For this review, take the finished solid that the model builds, in its own axes (mm). Face numbers are marked on the shaded views. A direction names the side the tool comes from. Coordinates: 2 decimals unless noted, no trailing zeros. Loops run counter-clockwise (first coordinate to the right, second up) from the corner with the lowest first, then second, coordinate; pieces in that order, holes last. Notation, with made-up numbers: (-28, -25.5) -> (-11, -25.5) arc R18 ccw to (-11, 7.5) -> close; hole circle Ø10 at (-1, 72.25). An arc over 180 degrees is marked (long way). Answer in a Markdown table with one row per item.
from build123d import *

# Parameters (mm, degrees)
Y_KSEKLIK_EKSTR_ZYON1_DEPTH = 12
Y_KSEKLIK_EKSTR_ZYON3_DEPTH = 15
KES_EKSTR_ZYON2_DEPTH       = 10
IZIM7_R                     = 3.5
KES_EKSTR_ZYON3_DEPTH       = 10
IZIM9_W                     = 16.31
IZIM9_H                     = 31
Y_KSEKLIK_EKSTR_ZYON4_DEPTH = 2
IZIM11_W                    = 16.312144578
IZIM11_H                    = 31
Y_KSEKLIK_EKSTR_ZYON5_DEPTH = 2
IZIM12_W                    = 16.312144578
IZIM12_H                    = 2
Y_KSEKLIK_EKSTR_ZYON6_DEPTH = 5
IZIM13_W                    = 16.31
IZIM13_H                    = 2
Y_KSEKLIK_EKSTR_ZYON7_DEPTH = 5
IZIM16_R                    = 1.5
KES_EKSTR_ZYON4_DEPTH       = 5


with BuildPart() as part:
    # Çizim1 → Yükseklik-Ekstrüzyon1 (new body)
    with BuildSketch(Plane(origin=(0, 0, 0), x_dir=(1, 0, 0), z_dir=(0, 1, 0))):
        with BuildLine():
            Line((-10.273080285, 9.233441174), (-24.270017386, 9.23050626))
            ThreePointArc((-24.270017386, 9.23050626), (-27.573247243, 1.740187513), (-24.270017386, -5.750131234))
            ThreePointArc((-24.270017386, -5.750131234), (-24.266862702, -5.754522055), (-24.265747955, -5.759812487))
            Line((-24.265747955, -5.759812487), (-10.280448773, -5.759812487))
            ThreePointArc((-10.280448773, -5.759812487), (-10.279708775, -5.756150024), (-10.277604879, -5.753062168))
            ThreePointArc((-10.277604879, -5.753062168), (-7.119784217, 1.739236804), (-10.273080285, 9.233441174))
        make_face()
    extrude(amount=Y_KSEKLIK_EKSTR_ZYON1_DEPTH)

    # Çizim2 → Yükseklik-Ekstrüzyon3 (add)
    with BuildSketch(Plane(origin=(0, 12, 0), x_dir=(1, 0, 0), z_dir=(0, 1, 0))):
        Polygon((-28.472879545, -6.371596623), (-24.972879545, -6.371596623), (-6.065973504, -6.371596623), (-6.065973504, 9.940547955), (-9.565973504, 9.940547955), (-28.472879545, 9.940547955), align=None)
        with BuildLine():
            ThreePointArc((-10.277604879, -5.753062168), (-10.279708775, -5.756150024), (-10.280448773, -5.759812487))
            Line((-10.280448773, -5.759812487), (-24.265747955, -5.759812487))
            ThreePointArc((-24.265747955, -5.759812487), (-24.266862702, -5.754522055), (-24.270017386, -5.750131234))
            ThreePointArc((-24.270017386, -5.750131234), (-27.573247243, 1.740187513), (-24.270017386, 9.23050626))
            Line((-24.270017386, 9.23050626), (-10.273080285, 9.233441174))
            ThreePointArc((-10.273080285, 9.233441174), (-7.119784217, 1.739236804), (-10.277604879, -5.753062168))
        make_face(mode=Mode.SUBTRACT)
    extrude(amount=-Y_KSEKLIK_EKSTR_ZYON3_DEPTH)

    # Çizim5 → Kes-Ekstrüzyon2 (cut)
    with BuildSketch(Plane(origin=(0, 0, 0), x_dir=(1, 0, 0), z_dir=(0, 1, 0))):
        with BuildLine():
            ThreePointArc((-24.253497742, -5.732043117), (-24.24760022, -5.74025453), (-24.24552089, -5.750148186))
            Line((-24.24552089, -5.750148186), (-10.281129786, -5.759812016))
            ThreePointArc((-10.281129786, -5.759812016), (-10.28107446, -5.75954361), (-10.280917812, -5.759318746))
            ThreePointArc((-10.280917812, -5.759318746), (-7.055942633, 1.738860839), (-10.261152425, 9.245510703))
            ThreePointArc((-10.261152425, 9.245510703), (-10.261308072, 9.245735025), (-10.261363099, 9.246002453))
            Line((-10.261363099, 9.246002453), (-24.245520899, 9.230533357))
            ThreePointArc((-24.245520899, 9.230533357), (-24.247598176, 9.220634198), (-24.253497742, 9.212418143))
            ThreePointArc((-24.253497742, 9.212418143), (-27.548750741, 1.740187513), (-24.253497742, -5.732043117))
        make_face()
    extrude(amount=KES_EKSTR_ZYON2_DEPTH, mode=Mode.SUBTRACT)

    # Çizim7 → Kes-Ekstrüzyon3 (cut)
    with BuildSketch(Plane(origin=(0, 12, 0), x_dir=(1, 0, 0), z_dir=(0, 1, 0))):
        with Locations((-17.269426524, 1.784475666)):
            Circle(IZIM7_R)
    extrude(amount=-KES_EKSTR_ZYON3_DEPTH, mode=Mode.SUBTRACT)

    # Çizim9 → Yükseklik-Ekstrüzyon4 (add)
    with BuildSketch(Plane.ZY.offset(28.472879545)):
        with Locations((-1.785547955, -3.5)):
            Rectangle(IZIM9_W, IZIM9_H)
    extrude(amount=Y_KSEKLIK_EKSTR_ZYON4_DEPTH)

    # Çizim11 → Yükseklik-Ekstrüzyon5 (add)
    with BuildSketch(Plane(origin=(-6.065973504, 0, 0), x_dir=(0, 0, -1), z_dir=(1, 0, 0))):
        with Locations((1.784475666, -3.5)):
            Rectangle(IZIM11_W, IZIM11_H)
    extrude(amount=Y_KSEKLIK_EKSTR_ZYON5_DEPTH)

    # Çizim12 → Yükseklik-Ekstrüzyon6 (add)
    with BuildSketch(Plane(origin=(-4.065973504, 0, 0), x_dir=(0, 0, -1), z_dir=(1, 0, 0))):
        with Locations((1.784475666, -18)):
            Rectangle(IZIM12_W, IZIM12_H)
    extrude(amount=Y_KSEKLIK_EKSTR_ZYON6_DEPTH)

    # Çizim13 → Yükseklik-Ekstrüzyon7 (add)
    with BuildSketch(Plane.ZY.offset(30.472879545)):
        with Locations((-1.785547955, -18)):
            Rectangle(IZIM13_W, IZIM13_H)
    extrude(amount=Y_KSEKLIK_EKSTR_ZYON7_DEPTH)

    # Çizim16 → Kes-Ekstrüzyon4 (cut)
    with BuildSketch(Plane.XZ.offset(19)):
        with Locations((-32.472879545, -1.785547955)):
            Circle(IZIM16_R)
        with Locations((-2.065973504, -1.784475666)):
            Circle(IZIM16_R)
    extrude(amount=-KES_EKSTR_ZYON4_DEPTH, mode=Mode.SUBTRACT)


solid = part.part
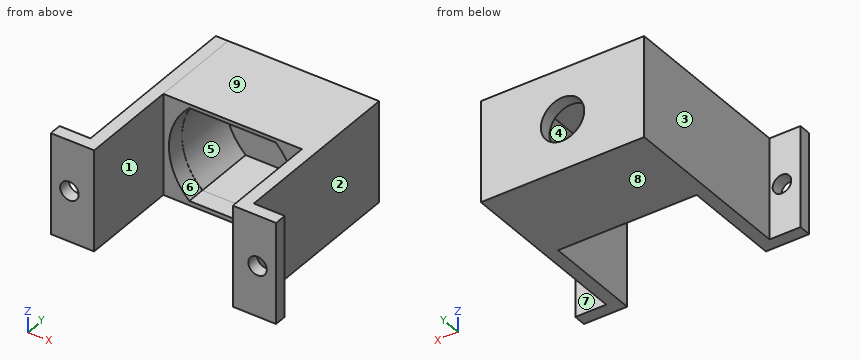
Item 1: Take a section at A-A, the plane y = -11.5. State the section outline as (x, z) points.
Worked answers:
| item | result |
|---|---|
| outline | (-30.47, -9.94) -> (-28.47, -9.94) -> (-28.47, 6.37) -> (-30.47, 6.37) -> close; (-6.07, -9.94) -> (-4.07, -9.94) -> (-4.07, 6.37) -> (-6.07, 6.37) -> close |
Item 2: For L1, parallel to X at y = -14, z = 4.25; L2, parallel to Z at x = -30, y = -1.5; L3, parallel to Y at x = -24, z = -1.25, list the stretches that pass through material, from the lowest coordinate up.
Worked answers:
| item | result |
|---|---|
| L1 | -30.47 to -28.47, -6.07 to -4.07 |
| L2 | -9.94 to 6.37 |
| L3 | 10 to 12 |
Item 3: Insertion check: pin 1 (6 mm diameter, centred on y = 6, z = 4.5, fed in from +X); pin 2 (8 mm diameter, centred on x = -11.5, z = -1.5, fed in from -Y); pin 3 (8 mm diameter, centred on y = -14, z = 1.5, fed in from -X); pin 4 (2.5 mm diameter, centred on x = -1.5, z = -1.5, fed in from +Y). Each pin has a flat end and moves straight along its axis. Give the tip position at first contact, or say it passes through.
Worked answers:
| item | result |
|---|---|
| pin 1 | x = -4.07 |
| pin 2 | y = 10 |
| pin 3 | x = -35.47 |
| pin 4 | y = -17 |
Item 4: For the marked faces 1, 2, 3, 4 and 5, list the 3-axis set-ups (+Z, -Z, +X, -X, +Y, -Y) from which the entire face can be reached by the end or side of a thin tool; tool diameter is ignored.
Worked answers:
| item | result |
|---|---|
| face 1 | +Z, -Z, -Y |
| face 2 | +Z, -Z, +X, +Y |
| face 3 | +Z, -Z, -X, +Y |
| face 4 | none |
| face 5 | -Y |
Item 5: The part is to be moulded in two halves that separate along Z. For the marked faces 6, 7, 8 and 9, say which applies: +Z half, -Z half, draft (parallel to the pull), parting line (faces both ways), or undercut.
Worked answers:
| item | result |
|---|---|
| face 6 | undercut |
| face 7 | draft |
| face 8 | -Z half |
| face 9 | +Z half |
